Can you work these out from the model? Positions are in its coordinate system, mm. A direction names the side the tool comes from. Coordinates: 2 decimals unless noted, no trailing zeros. Loops run counter-clockwise (first coordinate to the right, second up) from the corner with the lowest first, then second, coordinate; pieces in that order, holes last. Notation, with made-up numbers: M 88,85.25 L 122,85.25 A21 ccw 122,93.25 Z; hole C -9,-7.75 d8. An arc over 180 degrees is marked long. Return JSON: item names as keys, results as strings. Group by question number.
Autodesk Fusion 360 part; units mm, degrees
sketch "Esboço1" plane through (0, 0, 0) normal (0, 0, 1) x (1, 0, 0)
  line L0 (-0.023, -64.1886) -> (-14.118, -71.2361)
  arc A0 (-15.2361, -71.5) -> (-14.118, -71.2361) centre (-15.2361, -69) ccw
  line L1 (-15.2361, -71.5) -> (-42.5, -71.5)
  line L2 (-42.5, -71.5) -> (-45.5, -71.5)
  arc A1 (-45.5, -66.5) -> (-45.5, -71.5) centre (-45.5, -69) ccw
  arc A2 (-45.5, -66.5) -> (-42, -63) centre (-45.5, -63) ccw
  line L3 (-42, -63) -> (-42, -6)
  arc A3 (-39.5, -3.5) -> (-42, -6) centre (-39.5, -6) ccw
  line L4 (-39.5, -3.5) -> (-13, -3.5)
  line L5 (-9.5001, -3.5) -> (-13, -3.5)
  arc A4 (-9.5501, -8.4995) -> (-9.5001, -3.5) centre (-9.5001, -6) ccw
  line L6 (-9.5501, -8.4995) -> (-9.5966, -8.4995)
  arc A5 (-9.5966, -8.4995) -> (-13.0001, -11.9982) centre (-9.5001, -11.9982) ccw
  line L7 (-13.0001, -11.9982) -> (-13.0001, -47.0056)
  arc A6 (-13.0001, -47.0056) -> (-11.0979, -50.1196) centre (-9.5001, -47.0056) ccw
  line L8 (-11.0979, -50.1196) -> (-0.023, -55.8022)
  line L9 (-0.023, -64.1886) -> (-0.023, -55.8022)
extrude "Extrusão1" add sketch "Esboço1" along normal blind 1.8
sketch "Esboço2" plane through (0, 0, 1.8) normal (0, 0, 1) x (1, 0, 0)
  arc A0 (-15.2361, -71.5) -> (-14.118, -71.2361) centre (-15.2361, -69) ccw
  line L0 (-14.118, -71.2361) -> (-0.023, -64.1886)
  line L1 (-0.023, -64.1886) -> (-0.023, -55.8022)
  line L2 (-0.023, -55.8022) -> (-11.0979, -50.1196)
  arc A1 (-13.0001, -47.0056) -> (-11.0979, -50.1196) centre (-9.5001, -47.0056) ccw
  line L3 (-13.0001, -47.0056) -> (-13.0001, -11.9982)
  arc A2 (-9.5966, -8.4995) -> (-13.0001, -11.9982) centre (-9.5001, -11.9982) ccw
  line L4 (-9.5966, -8.4995) -> (-9.5501, -8.4995)
  arc A3 (-9.5501, -8.4995) -> (-9.5001, -3.5) centre (-9.5001, -6) ccw
  line L5 (-9.5001, -3.5) -> (-39.5, -3.5)
  arc A4 (-39.5, -3.5) -> (-42, -6) centre (-39.5, -6) ccw
  line L6 (-42, -6) -> (-42, -63)
  arc A5 (-45.5, -66.5) -> (-42, -63) centre (-45.5, -63) ccw
  arc A6 (-45.5, -66.5) -> (-45.5, -71.5) centre (-45.5, -69) ccw
  line L7 (-45.5, -71.5) -> (-42.5, -71.5)
  line L8 (-42.5, -71.5) -> (-15.2361, -71.5)
  circle A7 centre (-9.5001, -6) radius 0.75
  circle A8 centre (-45.5, -69) radius 0.75
  line L9 (-15.0001, -27.5) -> (-40.0001, -27.5)
  line L10 (-40.0001, -27.5) -> (-40.0001, -10.5)
  line L11 (-40.0001, -10.5) -> (-15.0001, -10.5)
  line L12 (-15.0001, -10.5) -> (-15.0001, -27.5)
  circle A9 centre (-30, -66) radius 1.5
  dimension "d10" = 1.5
  dimension "d11" = 1.5
  dimension "d12" = 25
  dimension "d13" = 17
  dimension "d14" = 2
  dimension "d15" = 1.9999
  dimension "d16" = 7
  dimension "d25" = 3
extrude "Extrusão2" cut sketch "Esboço2" against normal blind 4 contours A7 | A8 | L9 L10 L11 L12 | A9
chamfer "Chanfro1" distance 1.999 angle 30 4 edges at (-27.5001, -27.5, 1.8) (-40.0001, -19, 1.8) (-27.5001, -10.5, 1.8) (-15.0001, -19, 1.8) measured on face at (-27.7041, -46.3366, 1.8) measured on face at (-27.7041, -46.3366, 1.8) measured on face at (-27.7041, -46.3366, 1.8) measured on face at (-27.7041, -46.3366, 1.8)
fillet "Arredondamento1" radius 1.8 1 edges at (-0.023, -59.9954, 1.8)
chamfer "Chanfro2" distance 1 angle 45 2 edges at (-10.1993, -5.7288, 1.8) (-46.1992, -68.7288, 1.8) measured on face at (-28.3704, -47.0029, 1.8) measured on face at (-28.3704, -47.0029, 1.8)
chamfer "Chanfro3" distance 1.8 angle 45 1 edges at (-31.3985, -65.4576, 1.8) measured on face at (-28.3704, -47.0029, 1.8)
1) For pin 1 (0.7 mm diameter, centred on y = -21, z = 0, fed in from -X); pin 2 (0.5 mm diameter, centred on y = -24, z = 0.5, fed in from +X); pin 3 (1.7 mm diameter, centred on x = -9.5, y = -6, fed in from +Z), each with a flat end and sliding along its axis, tell me the tip position at first contact or that it passes through.
2) Suppose I cut it at A-A, the plane x = -30. Give the number of separate pieces and of enclosed holes in the cut face, then the cut area to 3 significant figures.
3) If we mould it in two halves opening along Y, with no side actions, what happens to faces 4 (the face through (-48, -69, 1)), 5 (the face through (-30, -71.5, 1)), 6 (the face through (-27.297, -9.514, 1.215))? For each: +Y half, -Y half, draft (parallel to the pull), parting line (faces both ways), or undercut.
4) Suppose I cut it at C-C, the plane x = -16.5. List the corners of the cut face in (y, z) for me.
5) Suppose I cut it at D-D, the plane z = 0.35. List the corners of the cut face in (x, y) for me, then the cut area to 3 significant figures.
6) For faces 1 (the face through (-40.986, -18.853, 1.215)), 2 (the face through (-25, -45, 1.8)), 3 (the face through (-12.473, -48.853, 0.887)), which set-ups out of +Z, -Z, +X, -X, +Y, -Y let a thin tool reach every point of the face, with its end or its side?
7) If I drill on line 1 (Y direction, x = -8.5, z = 1.55); line 2 (Y direction, x = -30.5, z = 1.55); line 3 (Y direction, x = -26, z = 0.25), over which ranges is the centre line in solid material (lowest first)? Write a range as from..to.
Returned:
{
 "1": {"pin 1": "stops at x = -42", "pin 2": "stops at x = -13", "pin 3": "stops at z = 0.9"},
 "2": {"separate pieces": "3", "enclosed holes": "0", "area": "80.9 mm²"},
 "3": {"face 4": "parting line", "face 5": "-Y half", "face 6": "undercut"},
 "4": {"outline": "M -71.5,0 L -27.5,0 L -27.5,0.65 L -29.5,1.8 L -71.5,1.8 Z; M -10.5,0 L -3.5,0 L -3.5,1.8 L -8.5,1.8 L -10.5,0.65 Z"},
 "5": {"outline": "M -45.5,-71.5 L -15.24,-71.5 A2.5 ccw -14.12,-71.24 L -0.06,-64.21 L -0.06,-55.78 L -11.1,-50.12 A3.5 cw -13,-47.01 L -13,-12 A3.5 cw -9.6,-8.5 L -9.55,-8.5 A2.5 ccw long -9.5,-3.5 L -39.5,-3.5 A2.5 ccw -42,-6 L -42,-63 A3.5 cw -45.5,-66.5 A2.5 ccw Z; hole C -45.5,-69 d1.5; hole M -40,-27.5 L -15,-27.5 L -15,-10.5 L -40,-10.5 Z; hole C -30,-66 d3.7; hole C -9.5,-6 d1.5", "area": "1,790 mm²"},
 "6": {"face 1": "+Z", "face 2": "+Z, +X, -X, +Y, -Y", "face 3": "+Z, -Z, +X"},
 "7": {"line 1": "y = -68.43..-51.45, -8.29..-7.12, -4.88..-3.71", "line 2": "y = -71.5..-69.01, -62.99..-29.07, -8.93..-3.5", "line 3": "y = -71.5..-27.5, -10.5..-3.5"}
}
